from build123d import *

# Parameters (mm, degrees)
SKETCH1_W                                  = 47.752
SKETCH1_H                                  = 71.816
BOSS_EXTRUDE1_DEPTH                        = 5
SKETCH2_W                                  = 38.608
SKETCH2_H                                  = 62.672
CUT_EXTRUDE1_DEPTH                         = 1.5
SKETCH3_W                                  = 4.064
SKETCH3_H                                  = 12.7
CUT_EXTRUDE2_DEPTH                         = 44.263123327
MIRROR4_AT_THE_SECOND_PLANE_COPY_1_SKETC_W = 4.064
MIRROR4_AT_THE_SECOND_PLANE_COPY_1_SKETC_H = 12.7
MIRROR4_AT_THE_SECOND_PLANE_COPY_1_DEPTH   = 44.263123327
FILLET2_R                                  = 1.5
SKETCH4_R                                  = 1.1303
CUT_EXTRUDE3_DEPTH                         = 44.263123327
MIRROR5_AT_THE_SECOND_PLANE_COPY_1_SKETC_R = 1.1303
MIRROR5_AT_THE_SECOND_PLANE_COPY_1_DEPTH   = 44.263123327
SKETCH5_W                                  = 38.608
SKETCH5_H                                  = 19.75
BOSS_EXTRUDE2_DEPTH                        = 1
CUT_EXTRUDE4_REACH                         = 45.41
MIRROR6_AT_THE_SECOND_PLANE_COPY_1_REACH   = 45.41


with BuildPart() as part:
    # Sketch1 → Boss-Extrude1 (new body)
    with BuildSketch(Plane(origin=(0, 0, 0), x_dir=(1, 0, 0), z_dir=(0, 1, 0))):
        Rectangle(SKETCH1_W, SKETCH1_H)
    extrude(amount=BOSS_EXTRUDE1_DEPTH)

    # Sketch2 → Cut-Extrude1 (cut)
    with BuildSketch(Plane(origin=(0, 5, 0), x_dir=(1, 0, 0), z_dir=(0, 1, 0))):
        Rectangle(SKETCH2_W, SKETCH2_H)
    extrude(amount=-CUT_EXTRUDE1_DEPTH, mode=Mode.SUBTRACT)

    # Sketch3 → Cut-Extrude2 (cut, through all)
    with BuildSketch(Plane(origin=(0, 3.5, 0), x_dir=(1, 0, 0), z_dir=(0, 1, 0))):
        with Locations((-17.272, 24.986)):
            Rectangle(SKETCH3_W, SKETCH3_H)
    cut_extrude2 = extrude(amount=-CUT_EXTRUDE2_DEPTH, mode=Mode.SUBTRACT)

    # Mirror4: Cut-Extrude2 across plane
    add(cut_extrude2.mirror(Plane.XY), mode=Mode.SUBTRACT)

    # Mirror4 at the second plane: Cut-Extrude2 across plane
    add(cut_extrude2.mirror(Plane(origin=(0, 0, 0), x_dir=(0, 0, 1), z_dir=(1, 0, 0))), mode=Mode.SUBTRACT)

    # Mirror4 at the second plane copy 1 sketc → Mirror4 at the second plane copy 1 (cut, through all)
    with BuildSketch(Plane(origin=(0, 3.5, 0), x_dir=(-1, 0, 0), z_dir=(0, 1, 0))):
        with Locations((-17.272, 24.986)):
            Rectangle(MIRROR4_AT_THE_SECOND_PLANE_COPY_1_SKETC_W, MIRROR4_AT_THE_SECOND_PLANE_COPY_1_SKETC_H)
    extrude(amount=-MIRROR4_AT_THE_SECOND_PLANE_COPY_1_DEPTH, mode=Mode.SUBTRACT)

    # Fillet2
    fillet2_edges = [part.edges().sort_by_distance(p)[0] for p in [
        (19.304, 2.5, -31.336),
        (19.304, 2.5, 31.336),
        (-19.304, 2.5, 31.336),
        (-19.304, 2.5, -31.336),
        (-19.304, 1.75, -18.636),
        (-15.24, 1.75, -31.336),
        (-15.24, 1.75, -18.636),
        (19.304, 1.75, -18.636),
        (15.24, 1.75, -18.636),
        (15.24, 1.75, -31.336),
        (-19.304, 1.75, 18.636),
        (-15.24, 1.75, 18.636),
        (-15.24, 1.75, 31.336),
        (19.304, 1.75, 18.636),
        (15.24, 1.75, 31.336),
        (15.24, 1.75, 18.636),
    ]]
    fillet(fillet2_edges, radius=FILLET2_R)

    # Sketch4 → Cut-Extrude3 (cut, through all)
    with BuildSketch(Plane(origin=(0, 3.5, 0), x_dir=(1, 0, 0), z_dir=(0, 1, 0))):
        with Locations(Location((-6.35, 27.907, 0), (0, 0, 270))):
            Circle(SKETCH4_R)
        with Locations(Location((-16.51, 15.842, 0), (0, 0, 270))):
            Circle(SKETCH4_R)
    cut_extrude3 = extrude(amount=-CUT_EXTRUDE3_DEPTH, mode=Mode.SUBTRACT)

    # Mirror5: Cut-Extrude3 across plane
    add(cut_extrude3.mirror(Plane.XY), mode=Mode.SUBTRACT)

    # Mirror5 at the second plane: Cut-Extrude3 across plane
    add(cut_extrude3.mirror(Plane(origin=(0, 0, 0), x_dir=(0, 0, 1), z_dir=(1, 0, 0))), mode=Mode.SUBTRACT)

    # Mirror5 at the second plane copy 1 sketc → Mirror5 at the second plane copy 1 (cut, through all)
    with BuildSketch(Plane(origin=(0, 3.5, 0), x_dir=(-1, 0, 0), z_dir=(0, 1, 0))):
        with Locations(Location((-6.35, 27.907, 0), (0, 0, 270))):
            Circle(MIRROR5_AT_THE_SECOND_PLANE_COPY_1_SKETC_R)
        with Locations(Location((-16.51, 15.842, 0), (0, 0, 270))):
            Circle(MIRROR5_AT_THE_SECOND_PLANE_COPY_1_SKETC_R)
    extrude(amount=-MIRROR5_AT_THE_SECOND_PLANE_COPY_1_DEPTH, mode=Mode.SUBTRACT)

    # Sketch5 → Boss-Extrude2 (add)
    with BuildSketch(Plane(origin=(0, 3.5, 0), x_dir=(1, 0, 0), z_dir=(0, 1, 0))):
        Rectangle(SKETCH5_W, SKETCH5_H)
    extrude(amount=BOSS_EXTRUDE2_DEPTH)

    # Cut-Extrude4: up to this face of the body (flat: up to its plane)
    cut_extrude4_end = Plane(part.part.faces().sort_by_distance((0, 3.5, -19.951636366))[0])
    # Sketch6 → Cut-Extrude4 (cut, up to the picked face)
    with BuildSketch(Plane(origin=(0, 5, 0), x_dir=(1, 0, 0), z_dir=(0, 1, 0)), mode=Mode.PRIVATE) as cut_extrude4_sk1:
        with BuildLine():
            Line((-19.304, 11.375), (-19.304, 9.875))
            ThreePointArc((-19.304, 9.875), (-20.054, 10.625), (-19.304, 11.375))
        make_face()
    cut_extrude4_tool1 = split(extrude(cut_extrude4_sk1.sketch, amount=-CUT_EXTRUDE4_REACH, mode=Mode.PRIVATE), bisect_by=cut_extrude4_end, keep=Keep.BOTH, mode=Mode.PRIVATE)
    cut_extrude4 = cut_extrude4_tool1.solids().sort_by(Axis((-19.62231, 5, -10.625), (0, -1, 0)))[0]
    add(cut_extrude4, mode=Mode.SUBTRACT)

    # Mirror6: Cut-Extrude4 across plane
    add(cut_extrude4.mirror(Plane.XY), mode=Mode.SUBTRACT)

    # Mirror6 at the second plane: Cut-Extrude4 across plane
    add(cut_extrude4.mirror(Plane(origin=(0, 0, 0), x_dir=(0, 0, 1), z_dir=(1, 0, 0))), mode=Mode.SUBTRACT)

    # Mirror6 at the second plane copy 1: up to this face of the body (flat: up to its plane)
    mirror6_at_the_second_plane_copy_1_end = Plane(part.part.faces().sort_by_distance((0, 3.5, 19.951636366))[0])
    # Mirror6 at the second plane copy 1 sketc → Mirror6 at the second plane copy 1 (cut, up to the picked face)
    with BuildSketch(Plane(origin=(0, 5, 0), x_dir=(-1, 0, 0), z_dir=(0, 1, 0)), mode=Mode.PRIVATE) as mirror6_at_the_second_plane_copy_1_sk1:
        with BuildLine():
            Line((-19.304, 11.375), (-19.304, 9.875))
            ThreePointArc((-19.304, 9.875), (-20.054, 10.625), (-19.304, 11.375))
        make_face()
    mirror6_at_the_second_plane_copy_1_tool1 = split(extrude(mirror6_at_the_second_plane_copy_1_sk1.sketch, amount=-MIRROR6_AT_THE_SECOND_PLANE_COPY_1_REACH, mode=Mode.PRIVATE), bisect_by=mirror6_at_the_second_plane_copy_1_end, keep=Keep.BOTH, mode=Mode.PRIVATE)
    add(mirror6_at_the_second_plane_copy_1_tool1.solids().sort_by(Axis((19.62231, 5, 10.625), (0, -1, 0)))[0], mode=Mode.SUBTRACT)


solid = part.part
Design review of the part built by this model. Coordinates are the model's own, in mm. A direction names the side the tool comes from. Round coordinates to 2 decimals unless told otherwise and drop trailing zeros. Write each loop counter-clockwise with the first axis right and the second up, starting at its lowest first coordinate (ties: lowest second). Pieces come first, ordered by that corner, then holes. Notation, with made-up numbers: (54, 1.5) - (68, 1.5) arc R14 cw to (68, 8.5) - close; hole circle Ø1 at (-6.75, 57). An arc over 180 degrees is marked (long way). Use a Markdown table: item, result. Add a question column.
1. We need section C-C (x = 12.5). State the section outline as (y, z) points (3 decimals), then the cut area to 3 significant figures.
2. We need section B-B (y = 0.7). Count the separate pieces of the cut face and the enclosed holes in it, then the cut area to 3 significant figures.
3. Wall thickness on probe 1 along Z at (x, y) = (16.51, 1.4); probe 2 along X at (y, z) = (2.15, -16); probe 3 along X at (y, z) = (0.55, 21): over which ranges is each line inside the solid? List them lowest first.
4. We need section A-A (x = 6.35). State the section outline as (y, z) points (3 decimals), then the cut area to 3 significant figures.
5. Clearance check with flat-ended pins moving along their axes: pin 1 (2 mm diameter, centred on x = 16.51, z = 15.842, fed in from -Y); pin 2 (3 mm diameter, centred on x = 6.35, z = 27.907, fed in from +Y); pin 3 (2.5 mm diameter, centred on x = -6.35, z = 27.907, fed in from -Y). State where each tip first meets the part, or that it passes through.
6. For faces 1 (the face through (-20.054, 4.26, -10.609)), 2 (the face through (-18.88, 1.73, 19.09)), list the 3-axis set-ups (+Z, -Z, +X, -X, +Y, -Y) from which the entire face can be reached by the end or side of a thin tool; tool diameter is ignored.
Output:
| question | item | result |
|---|---|---|
| 1 | outline | (0, -35.908) - (5, -35.908) - (5, -31.336) - (3.5, -31.336) - (3.5, -9.875) - (4.5, -9.875) - (4.5, 9.875) - (3.5, 9.875) - (3.5, 31.336) - (5, 31.336) - (5, 35.908) - (0, 35.908) - close |
| 1 | area | 285 mm2 |
| 2 | separate pieces | 1 |
| 2 | enclosed holes | 12 |
| 2 | area | 3,200 mm2 |
| 3 | probe 1 | z = -35.91 to -31.32, -18.65 to -16.97, -14.71 to 14.71, 16.97 to 18.65, 31.32 to 35.91 |
| 3 | probe 2 | x = -23.88 to -17.63, -15.39 to 15.39, 17.63 to 23.88 |
| 3 | probe 3 | x = -23.88 to -19.3, -15.24 to 15.24, 19.3 to 23.88 |
| 4 | outline | (0, -35.908) - (5, -35.908) - (5, -31.336) - (3.5, -31.336) - (3.5, -29.037) - (0, -29.037) - close; (0, -26.777) - (3.5, -26.777) - (3.5, -9.875) - (4.5, -9.875) - (4.5, 9.875) - (3.5, 9.875) - (3.5, 26.777) - (0, 26.777) - close; (0, 29.037) - (3.5, 29.037) - (3.5, 31.336) - (5, 31.336) - (5, 35.908) - (0, 35.908) - close |
| 4 | area | 269 mm2 |
| 5 | pin 1 | passes through |
| 5 | pin 2 | stops at y = 3.5 |
| 5 | pin 3 | stops at y = 0 |
| 6 | face 1 | +Y |
| 6 | face 2 | +Y, -Y |
